from build123d import *

# Parameters (mm, degrees)
SKETCH_R        = 10.5
PAD_DEPTH       = 15
POCKET_DEPTH    = 7
SKETCH002_R     = 5.5
POCKET001_DEPTH = 6.5
CHAMFER_SIZE    = 2


with BuildPart() as part:
    # Sketch → Pad (new body)
    with BuildSketch(Plane.XY):
        Circle(SKETCH_R)
    extrude(amount=PAD_DEPTH)

    # Sketch001 (on Face3 of Pad) → Pocket (cut)
    with BuildSketch(Plane.XY.offset(15)):
        Polygon((6.920429, -4.179273), (7.079571, 3.903631), (0.159142, 8.082904), (-6.920429, 4.179273), (-7.079571, -3.903631), (-0.159142, -8.082904), align=None)
    extrude(amount=-POCKET_DEPTH, mode=Mode.SUBTRACT)

    # Sketch002 (on Face10 of Pocket) → Pocket001 (cut)
    with BuildSketch(Plane.XY.offset(8)):
        Circle(SKETCH002_R)
    extrude(amount=-POCKET001_DEPTH, mode=Mode.SUBTRACT)

    # Chamfer
    chamfer_edges = [part.edges().sort_by_distance(p)[0] for p in [
        (-10.5, 0, 0),
    ]]
    chamfer(chamfer_edges, length=CHAMFER_SIZE)


solid = part.part
Check sheet for the modelled part. Datum: model origin and axes. Units: mm. A direction names the side the tool comes from. Round coordinates to 2 decimals unless told otherwise and drop trailing zeros. Order: outer loops, then holes, each group sorted by start corner. A loop starts at its lowest first (then second) coordinate and runs counter-clockwise, first axis right, second up. Notation, with made-up numbers: M -32.5,-34 L -2.5,-34 A20 ccw -2.5,-29 Z; hole C 71,-4 d10. An arc over 180 degrees is marked long. One line per item, written item: value. Start each with the question number.
1. Scan lines: line 1 along Y through (x, z) = (0, 6); line 2 along Y through (x, z) = (-7.75, 10.75); line 3 along Z through (x, y) = (1.75, 3). Record each from-to range of solid material in increasing order.
2. Release check for a two-part mould opening along Y. For faces 3 (the cylindrical face through (10, 3.2, 8.4)), 4 (the flat face through (0, 0, 0)), 5 (the flat face through (-3, 5, 8)) record: released by +Y, released by -Y, zero draft, split by the parting line, or undercut.
3. Section check A-A on z = 8.5. Enter the section's corners in (x, y), and give its area (3 significant figures).
4. Section check C-C on z = 4.5. Enter the section's corners in (x, y).
5. Gauge pin test, flat ends, axial feed: P1, Ø4, axis at x = 1, y = -1.5, coming from the +Z side; P2, Ø5, axis at y = -7, z = 8, coming from the -X side; P3, Ø9, axis at x = 2, y = 1, coming from the +Z side. Record the tip position at first contact, or that the pin passes through.
6. Section check B-B on y = 0. Enter the section's corners in (x, z), and give its area (3 significant figures).
7. Access from +Z, -Z, +X, -X, +Y, -Y to the whole of each face (thin tool, end or side, straight path). Record for faces 1 (the flat face through (3.33, -6.16, 11.55)), 2 (the flat face through (-2.5, -6.9, 15)).
Results found:
1. line 1: -10.5 to -5.5, 5.5 to 10.5
1. line 2: -7.08 to 7.08
1. line 3: 0 to 1.5
2. face 3: split by the parting line
2. face 4: zero draft
2. face 5: undercut
3. outline: C 0,0 d21; hole M -7.08,-3.9 L -0.16,-8.08 L 6.92,-4.18 L 7.08,3.9 L 0.16,8.08 L -6.92,4.18 Z
3. area: 177 mm^2
4. outline: C 0,0 d21; hole C 0,0 d11
5. P1: z = 1.5
5. P2: x = -9.49
5. P3: z = 8
6. outline: M -10.5,2 L -8.5,0 L 8.5,0 L 10.5,2 L 10.5,15 L 7,15 L 7,8 L 5.5,8 L 5.5,1.5 L -5.5,1.5 L -5.5,8 L -7,8 L -7,15 L -10.5,15 Z
6. area: 141 mm^2
7. face 1: +Z
7. face 2: +Z, +X, -X, +Y, -Y
